Design review of the part built by this model. Coordinates are the model's own, in mm. A direction names the side the tool comes from. Coordinates: 2 decimals unless noted, no trailing zeros. Write each loop counter-clockwise with the first axis right and the second up, starting at its lowest first coordinate (ties: lowest second). Pieces come first, ordered by that corner, then holes. Notation, with made-up numbers: (39, 9.5) -> (62, 9.5) arc R13 ccw to (62, 13.5) -> close; hole circle Ø10 at (75, -21). An arc over 180 degrees is marked (long way). One line per question, with ' | ' between items. Start each with the question number.
Q1. Wall thickness on probe 1 along Y at (x, z) = (5.25, 9.75); probe 2 along Y at (x, z) = (3.75, 12.25); probe 3 along X at (y, z) = (22.7, 2.05): over which ranges is each line inside the solid? List them lowest first.
Q2. Add section A-A on z = 2.5. State the section outline as (x, y) points.
Q3. Add section B-B on y = 22.7. State the section outline as (x, z) points.
Q4. Draft analysis for pull direction X (two halves, no side actions). For faces 1 (the cylindrical face through (13.675, 45.099, 0.285)), 2 (the cylindrical face through (26.715, 0.301, 4.802)), 3 (the flat face through (5.4, 41, 12)), state which applies: pulls with the +X half, pulls with the -X half, needs draft (parallel to the pull), parting line crosses it, or undercut.
Q5. For P1, Ø1, axis at x = 15.5, y = 40.5, coming from the +Z side; P2, Ø0.9, axis at x = 24.5, z = 4.5, coming from the +Y side; P3, Ø5, axis at y = 45, z = 19.5, coming from the -X side; P4, Ø4.5, axis at y = 0.5, z = 10.5, coming from the +X side, all flat-tipped, find the tip position at first contact; note any pin that passes through.
Q6. For faces 4 (the flat face through (9.5, 44, 20)), 5 (the flat face through (25, 5, 15)), 6 (the flat face through (4, 5, 21.5)), 7 (the flat face through (7, 2, 6)), list the 3-axis set-ups (+Z, -Z, +X, -X, +Y, -Y) from which the entire face can be reached by the end or side of a thin tool; tool diameter is ignored.
Q7. Add section C-C on x = 13.5. State the section outline as (y, z) points, and give its area (3 significant figures).
Q8. Add section D-D on y = 35. State the section outline as (x, z) points, and give its area (3 significant figures).
from build123d import *

# Parameters (mm, degrees)
SKETCH_1_W           = 27
SKETCH_1_H           = 45.4
SKETCH_1_R           = 6.5
EXTRUDE_1_DEPTH      = 8.5
CUT_EXTRUDE_1_DEPTH  = 21
SKETCH_3_W           = 23
SKETCH_3_H           = 41.4
CUT_EXTRUDE_2_DEPTH  = 5.5
EXTRUDE_2_DEPTH      = 18.5
EXTRUDE_3_DEPTH      = 5.25
EXTRUDE_3_DEPTH_BACK = 5.25
SKETCH_7_W           = 4
SKETCH_7_H           = 1
SKETCH_7_W_2         = 7
CUT_EXTRUDE_3_DEPTH  = 3
SKETCH_8_W           = 7
SKETCH_8_H           = 1
SKETCH_8_W_2         = 4
CUT_EXTRUDE_4_DEPTH  = 3
CUT_EXTRUDE_START    = -15.5
SKETCH_9_W           = 8
SKETCH_9_H           = 13.007388574
CUT_EXTRUDE_5_DEPTH  = 15.5
FILLET_1_R           = 1
FILLET_3_R           = 1
SKETCH_10_W          = 22.881985058
SKETCH_10_H          = 38.494603021
SKETCH_10_R          = 6.5
EXTRUDE_4_DEPTH      = 3


with BuildPart() as part:
    # Эскиз1 → Бобышка-Вытянуть1 (new body)
    with BuildSketch(Plane.XY):
        with Locations((13.5, 22.7)):
            Rectangle(SKETCH_1_W, SKETCH_1_H)
        with Locations((13.5, 22.7)):
            Circle(SKETCH_1_R, mode=Mode.SUBTRACT)
    extrude(amount=EXTRUDE_1_DEPTH)

    # Эскиз2 → Вырез-Вытянуть1 (cut)
    with BuildSketch(Plane(origin=(3, 0, 0), x_dir=(0, 0, -1), z_dir=(1, 0, 0))):
        with BuildLine():
            Line((0, 40.4), (0, 5))
            ThreePointArc((0, 5), (-1, 22.7), (0, 40.4))
        make_face()
    extrude(amount=CUT_EXTRUDE_1_DEPTH, mode=Mode.SUBTRACT)

    # Эскиз3 → Вырез-Вытянуть2 (cut)
    with BuildSketch(Plane.XY.offset(8.5)):
        with Locations((13.5, 22.7)):
            Rectangle(SKETCH_3_W, SKETCH_3_H)
    extrude(amount=-CUT_EXTRUDE_2_DEPTH, mode=Mode.SUBTRACT)

    # Эскиз4 → Бобышка-Вытянуть2 (add)
    with BuildSketch(Plane.XY.offset(3)):
        Polygon((3.8, 45.4), (3.8, 41.4), (2, 41.4), (2, 39.8), (3.8, 39.8), (3.8, 36.4), (5.4, 36.4), (5.4, 45.4), align=None)
        Polygon((21.6, 45.4), (23.2, 45.4), (23.2, 41.4), (25, 41.4), (25, 39.8), (23.2, 39.8), (23.2, 36.4), (21.6, 36.4), align=None)
        Polygon((23.2, 0), (23.2, 4), (25, 4), (25, 5.6), (23.2, 5.6), (23.2, 9), (21.6, 9), (21.6, 0), align=None)
        Polygon((5.4, 0), (3.8, 0), (3.8, 4), (2, 4), (2, 5.6), (3.8, 5.6), (3.8, 9), (5.4, 9), align=None)
    extrude(amount=EXTRUDE_2_DEPTH)

    # Эскиз6 → Бобышка-Вытянуть3 (add, two sides: drawn at the far end of the back side and taken through both)
    with BuildSketch(Plane.ZY.offset(-13.5).offset(-EXTRUDE_3_DEPTH_BACK)):
        Polygon((3, 2), (3, 3.6), (24, 3.6), (24, 2), (17, -2.3), (15, 2), align=None)
        Polygon((18, 43.4), (3, 43.4), (3, 41.8), (24, 41.8), (24, 43.4), (20, 47.7), align=None)
    extrude(amount=EXTRUDE_3_DEPTH + EXTRUDE_3_DEPTH_BACK)

    # Эскиз7 → Вырез-Вытянуть3 (cut)
    with BuildSketch(Plane.ZY.offset(-3.8)):
        with Locations((19.5, 44.9)):
            Rectangle(SKETCH_7_W, SKETCH_7_H)
        with Locations((18, 0.5)):
            Rectangle(SKETCH_7_W_2, SKETCH_7_H)
    extrude(amount=-CUT_EXTRUDE_3_DEPTH, mode=Mode.SUBTRACT)

    # Эскиз8 → Вырез-Вытянуть4 (cut)
    with BuildSketch(Plane(origin=(23.2, 0, 0), x_dir=(0, 0, -1), z_dir=(1, 0, 0))):
        with Locations((-18, 0.5)):
            Rectangle(SKETCH_8_W, SKETCH_8_H)
        with Locations((-19.5, 44.9)):
            Rectangle(SKETCH_8_W_2, SKETCH_8_H)
    extrude(amount=-CUT_EXTRUDE_4_DEPTH, mode=Mode.SUBTRACT)

    # Эскиз9 → Вырез-Вытянуть5 (cut)
    with BuildSketch(Plane.XY.offset(24).offset(CUT_EXTRUDE_START)):
        with Locations((13.5, -4.103694287)):
            Rectangle(SKETCH_9_W, SKETCH_9_H)
        with Locations((13.5, 49.503694287)):
            Rectangle(SKETCH_9_W, SKETCH_9_H)
    extrude(amount=CUT_EXTRUDE_5_DEPTH, mode=Mode.SUBTRACT)

    # Скругление1
    fillet_1_edges = [part.edges().sort_by_distance(p)[0] for p in [
        (13.5, 45.4, 0),
        (27, 22.7, 0),
        (13.5, 0, 0),
        (0, 22.7, 0),
        (0, 45.4, 4.25),
        (27, 45.4, 4.25),
        (27, 0, 4.25),
        (0, 0, 4.25),
    ]]
    fillet(fillet_1_edges, radius=FILLET_1_R)

    # Скругление3
    fillet_3_edges = [part.edges().sort_by_distance(p)[0] for p in [
        (8.875, 2, 8.5),
        (18.75, 2.8, 3),
        (13.5, 3.6, 3),
        (8.25, 2.8, 3),
        (18.125, 43.4, 8.5),
        (13.5, 41.8, 3),
        (18.75, 42.6, 3),
        (8.25, 42.6, 3),
    ]]
    fillet(fillet_3_edges, radius=FILLET_3_R)

    # Эскиз10 → Бобышка-Вытянуть4 (add)
    with BuildSketch(Plane(origin=(0, 0, 0), x_dir=(-1, 0, 0), z_dir=(0, 0, -1))):
        with Locations((-13.488807008, 22.65959588)):
            Rectangle(SKETCH_10_W, SKETCH_10_H)
        with Locations((-13.5, 22.7)):
            Circle(SKETCH_10_R, mode=Mode.SUBTRACT)
    extrude(amount=-EXTRUDE_4_DEPTH)


solid = part.part
Output values:
1) probe 1: y = 0 to 9, 36.4 to 45.4 | probe 2: y = 4 to 5.6, 39.8 to 41.4 | probe 3: x = 0 to 7, 20 to 27
2) outline: (0, 1) arc R1 ccw to (1, 0) -> (26, 0) arc R1 ccw to (27, 1) -> (27, 44.4) arc R1 ccw to (26, 45.4) -> (1, 45.4) arc R1 ccw to (0, 44.4) -> close; hole circle Ø13 at (13.5, 22.7)
3) outline: (0, 1) arc R1 ccw to (1, 0) -> (7, 0) -> (7, 3) -> (2, 3) -> (2, 8.5) -> (0, 8.5) -> close; (20, 0) -> (26, 0) arc R1 ccw to (27, 1) -> (27, 8.5) -> (25, 8.5) -> (25, 3) -> (20, 3) -> close
4) face 1: needs draft | face 2: pulls with the +X half | face 3: undercut
5) P1: stops at z = 3.02 | P2: stops at y = 45.4 | P3: stops at x = 3.8 | P4: stops at x = 27
6) face 4: +Z, +Y | face 5: +Z, +X, +Y, -Y | face 6: +Z, -X, +Y, -Y | face 7: +Z
7) outline: (0, 1) arc R1 ccw to (1, 0) -> (16.2, 0) -> (16.2, 3) -> (4.6, 3) arc R1 cw to (3.6, 4) -> (3.6, 24) -> (2.4, 24) -> (2.4, 8.5) -> (0, 8.5) -> close; (29.2, 0) -> (44.4, 0) arc R1 ccw to (45.4, 1) -> (45.4, 8.5) -> (43, 8.5) -> (43, 24) -> (41.8, 24) -> (41.8, 4) arc R1 cw to (40.8, 3) -> (29.2, 3) -> close | area: 174 mm2
8) outline: (0, 1) arc R1 ccw to (1, 0) -> (26, 0) arc R1 ccw to (27, 1) -> (27, 8.5) -> (25, 8.5) -> (25, 3) -> (2, 3) -> (2, 8.5) -> (0, 8.5) -> close | area: 103 mm2
